Model file for the job. Use its own axes, mm. Round coordinates to 2 decimals unless told otherwise and drop trailing zeros. Order: outer loops, then holes, each group sorted by start corner. A loop starts at its lowest first (then second) coordinate and runs counter-clockwise, first axis right, second up. Notation, with made-up numbers: M 11.25,-16 L 61.25,-16 A6 ccw 61.25,-8 Z; hole C 89,32 d8. An arc over 180 degrees is marked long. Return JSON: item names as keys, results as strings. Group by question number.
Item 1: Slice it at A-A on z = 47.5. Write the cut outline in (x, y) (3 decimals), then the cut area to 3 significant figures.
Item 2: Pin check, flat tips, straight feed: pin 1 Ø1.6 at (y, z) = (-1.5, -57) entering from -X (3 decimals); pin 2 Ø1 at (y, z) = (-1.5, -48) entering from +X (3 decimals). Stop position of each tip, or through.
Item 3: Probe line 1 along X through (y, z) = (-2.25, 53.5) (3 decimals). List the from-to ranges inside material, lowest first.
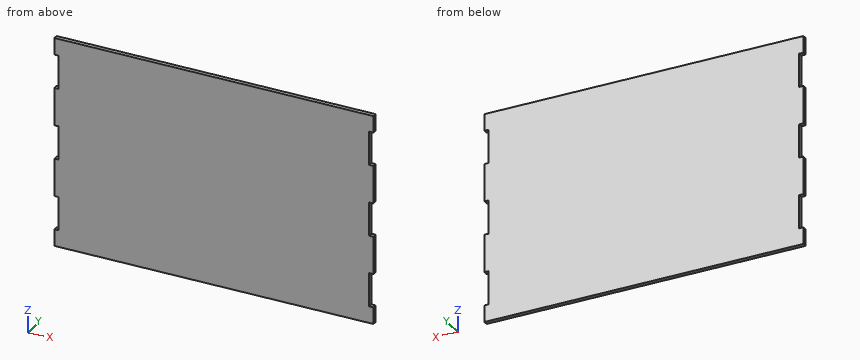
from build123d import *

# Parameters (mm, degrees)
F1_DEPTH = 3.175


with BuildPart() as f1:
    # F0 (on Front) → F1 (new body)
    with BuildSketch(Plane.XZ):
        Polygon((-120.65, -79.375), (120.65, -79.375), (120.65, -66.675), (117.475, -66.675), (117.475, -41.275), (120.65, -41.275), (120.65, -12.7), (117.475, -12.7), (117.475, 0), (117.475, 12.7), (120.65, 12.7), (120.65, 41.275), (117.475, 41.275), (117.475, 66.675), (120.65, 66.675), (120.65, 79.375), (-120.65, 79.375), (-120.65, 66.675), (-117.475, 66.675), (-117.475, 41.275), (-120.65, 41.275), (-120.65, 12.7), (-117.475, 12.7), (-117.475, 0), (-117.475, -12.7), (-120.65, -12.7), (-120.65, -41.275), (-117.475, -41.275), (-117.475, -66.675), (-120.65, -66.675), align=None)
    extrude(amount=F1_DEPTH)


solid = f1.part
Output values:
{
 "1": {"outline": "M -117.475,-3.175 L 117.475,-3.175 L 117.475,0 L -117.475,0 Z", "area": "746 mm²"},
 "2": {"pin 1": "x = -117.475", "pin 2": "x = 117.475"},
 "3": {"line 1": "-117.475 to 117.475"}
}
